```python
from build123d import *

# Parameters (mm, degrees)
F0_R     = 10
F1_DEPTH = 15
F3_DEPTH = 10


with BuildPart() as f1:
    # F0 (on Front) → F1 (new body)
    with BuildSketch(Plane.XZ):
        with BuildLine():
            ThreePointArc((0, -50), (10.606602, -45.606602), (15, -35))
            Line((15, -35), (15, 35))
            ThreePointArc((15, 35), (10.606602, 45.606602), (0, 50))
            ThreePointArc((0, 50), (-10.606602, 45.606602), (-15, 35))
            Line((-15, 35), (-15, -35))
            ThreePointArc((-15, -35), (-10.606602, -45.606602), (0, -50))
        make_face()
        with Locations((0, -35)):
            Circle(F0_R, mode=Mode.SUBTRACT)
    extrude(amount=F1_DEPTH)

    # F2 (on Front) → F3 (join)
    with BuildSketch(Plane.XZ):
        with BuildLine():
            ThreePointArc((0, 40), (-3.535534, 31.464466), (5, 35))
            ThreePointArc((5, 35), (3.535534, 38.535534), (0, 40))
        make_face()
    extrude(amount=-F3_DEPTH)


solid = f1.part
```
For this review, take the finished solid that the model builds, in its own axes (mm). Round coordinates to 2 decimals unless told otherwise and drop trailing zeros. Write each loop counter-clockwise with the first axis right and the second up, starting at its lowest first coordinate (ties: lowest second). Pieces come first, ordered by that corner, then holes.
1) Take a section at A-A on y = -2.5. Give the boundary of the cut face in (x, z), then the cut area to 3 significant figures.
Answer below:
outline: (-15, -35) arc R15 ccw to (0, -50) arc R15 ccw to (15, -35) - (15, 35) arc R15 ccw to (0, 50) arc R15 ccw to (-15, 35) - close; hole circle Ø20 at (0, -35)
area: 2,490 mm2
2) Take a section at C-C on x = -4. Give the boundary of the cut face in (y, z), then the cut area to 3 significant figures.
Answer below:
outline: (-15, -49.46) - (0, -49.46) - (0, -44.17) - (-15, -44.17) - close; (-15, -25.83) - (0, -25.83) - (0, 32) - (10, 32) - (10, 38) - (0, 38) - (0, 49.46) - (-15, 49.46) - close
area: 1,270 mm2
3) For line 1 along Y through (x, z) = (-8.5, -45.5); line 2 along Z through (x, y) = (1, -10); line 3 along Z through (x, y) = (4.5, -5.5), list the stretches that pass through material, from the lowest coordinate up.
Answer below:
line 1: y = -15 to 0
line 2: z = -49.97 to -44.95, -25.05 to 49.97
line 3: z = -49.31 to -43.93, -26.07 to 49.31
4) Take a section at B-B on z = -44. Give the boundary of the cut face in (x, y), then the cut area to 3 significant figures.
Answer below:
outline: (-12, -15) - (-4.36, -15) - (-4.36, 0) - (-12, 0) - close; (4.36, -15) - (12, -15) - (12, 0) - (4.36, 0) - close
area: 229 mm2
5) Take a section at D-D on y = 3.5. Give the boundary of the cut face in (x, z).
Answer below:
outline: circle Ø10 at (0, 35)
6) Insertion check: pin 1 Ø4 at (x, z) = (6.5, 1.5) entering from +Y; pin 2 Ø8 at (x, y) = (9, -6) entering from +Z; pin 3 Ø4 at (x, z) = (-7.5, -36.5) entering from +Y. Each pin has a flat end and moves straight along its axis. Give the tip position at first contact, or say it passes through.
Answer below:
pin 1: stops at y = 0
pin 2: stops at z = 49.14
pin 3: passes through
7) Mouldability with a two-part tool opening along X and no side actions: class faces 1 (the face through (0, 0, 1)), 2 (the face through (-15, -7, 0)), 3 (the face through (-2.17, -7.4, -44.76)) as +X half, -X half, draft (parallel to the pull), parting line (faces both ways), or undercut.
Answer below:
face 1: draft
face 2: -X half
face 3: undercut
